from build123d import *

# Parameters (mm, degrees)
SKETCH1_W           = 12.5
SKETCH1_H           = 5.7
BOSS_EXTRUDE1_DEPTH = 6.4
BOSS_EXTRUDE2_DEPTH = 5.7
SKETCH3_R           = 0.3
BOSS_EXTRUDE3_DEPTH = 3.5
SKETCH4_R           = 1
CUT_EXTRUDE1_DEPTH  = 1


with BuildPart() as part:
    # Sketch1 → Boss-Extrude1 (new body)
    with BuildSketch(Plane(origin=(0, 0, 0), x_dir=(1, 0, 0), z_dir=(0, 1, 0))):
        with Locations((1.136363636, 0.50625)):
            Rectangle(SKETCH1_W, SKETCH1_H)
    extrude(amount=BOSS_EXTRUDE1_DEPTH)

    # Sketch2 → Boss-Extrude2 (add)
    with BuildSketch(Plane.XY.offset(2.34375)):
        Polygon((-5.113636364, 6.4), (8.986363636, 10.3), (8.986363636, 10.092490462), (-5.113636364, 6.192490462), align=None)
    extrude(amount=-BOSS_EXTRUDE2_DEPTH)

    # Sketch3 → Boss-Extrude3 (add)
    with BuildSketch(Plane.XZ):
        with Locations(Location((-3.513636364, -0.50625, 0), (0, 0, 90))):
            Circle(SKETCH3_R)
        with Locations(Location((1.136363636, -0.50625, 0), (0, 0, 90))):
            Circle(SKETCH3_R)
        with Locations(Location((5.786363636, -0.50625, 0), (0, 0, 90))):
            Circle(SKETCH3_R)
    extrude(amount=BOSS_EXTRUDE3_DEPTH)

    # Sketch4 → Cut-Extrude1 (cut)
    with BuildSketch(Plane(origin=(0, 6.4, 0), x_dir=(1, 0, 0), z_dir=(0, 1, 0))):
        with Locations(Location((5.786363636, 0.50625, 0), (0, 0, 270))):
            Circle(SKETCH4_R)
    extrude(amount=-CUT_EXTRUDE1_DEPTH, mode=Mode.SUBTRACT)


solid = part.part
Source: CAD feature listing. Evaluate the final solid. Frame: model axes, mm. A direction names the side the tool comes from. Give positions to 0.01 mm unless a question says otherwise; leave off trailing zeros. Write each loop counter-clockwise with the first axis right and the second up, starting at its lowest first coordinate (ties: lowest second). Pieces come first, ordered by that corner, then holes. Notation, with made-up numbers: (83.5, 76.5) - (88.5, 76.5) arc R31 ccw to (88.5, 101.5) - close; hole circle Ø10 at (21.5, 6.5). An arc over 180 degrees is marked (long way). Write item = value, one per line. Start each with the question number.
Q1. Cut plane C-C, the plane y = -0.25. Return loops of the section in (x, z), then the cut area to 3 significant figures.
Q2. Pin query (flat end, axial travel): pin 1 Ø1.5 at (x, z) = (7.5, -1.5) entering from -Y; pin 2 Ø3 at (y, z) = (2, -0.5) entering from +X; pin 3 Ø1.7 at (x, z) = (3.5, 0) entering from +Y. Return the tip coordinate at first contact, or that it passes through.
Q3. Cut plane A-A, the plane z = 1.75. Return loops of the section in (x, y).
Q4. Cut plane D-D, the plane z = 0. Return loops of the section in (x, y), then the cut area to 3 significant figures.
Q5. Material intervals for probe 1 along X at (y, z) = (-3, -0.35); probe 2 along X at (y, z) = (3, -1); probe 3 along Y at (x, z) = (6.75, 1.45), sorted ascending.
Q6. Draft query along Z for faces 6 (the flat face through (1, 0, 0)), 7 (the flat face through (2, 4, -3.356)), 8 (the flat face through (6, 5.4, -1)). Return one class per face: +Z half, -Z half, draft (parallel to the pull), parting line (faces both ways), or undercut.
Q7. Cut plane B-B, the plane x = -2. Return loops of the section in (y, z).
Q8. Reachability of faces 1 (the flat face through (1.838, 8.323, -0.466)), 2 (the cylindrical face through (6.778, 5.907, -0.636)), 3 (the flat face through (7.386, 3, 0)), 4 (the flat face through (-5.114, 3, 0)), 5 (the flat face through (1, 6.4, -1)) from +Z, -Z, +X, -X, +Y, -Y: full face, straight path, thin tool, end or side. Return the list, or none.
Computed values:
q1.outline = circle Ø0.6 at (-3.51, -0.51); circle Ø0.6 at (1.14, -0.51); circle Ø0.6 at (5.79, -0.51)
q1.area = 0.848 mm²
q2.pin_1 = 0
q2.pin_2 = 7.39
q2.pin_3 = 9.02
q3.outline = (-5.11, 0) - (7.39, 0) - (7.39, 6.4) - (-4.36, 6.4) - (8.99, 10.09) - (8.99, 10.3) - (-5.11, 6.4) - close
q4.outline = (-5.11, 0) - (7.39, 0) - (7.39, 6.4) - (6.65, 6.4) - (6.65, 5.4) - (4.92, 5.4) - (4.92, 6.4) - (-4.36, 6.4) - (8.99, 10.09) - (8.99, 10.3) - (-5.11, 6.4) - close
q4.area = 81.1 mm²
q5.probe_1 = -3.77 to -3.26, 0.88 to 1.39, 5.53 to 6.04
q5.probe_2 = -5.11 to 7.39
q5.probe_3 = 0 to 6.4, 9.47 to 9.68
q6.face_6 = draft
q6.face_7 = -Z half
q6.face_8 = undercut
q7.outline = (0, -3.36) - (6.4, -3.36) - (6.4, 2.34) - (0, 2.34) - close; (7.05, -3.36) - (7.26, -3.36) - (7.26, 2.34) - (7.05, 2.34) - close
q8.face_1 = +Z, -Z, -X, +Y
q8.face_2 = none
q8.face_3 = +Z, -Z, +X, -Y
q8.face_4 = +Z, -Z, -X, +Y, -Y
q8.face_5 = +Z, -Z, +X
